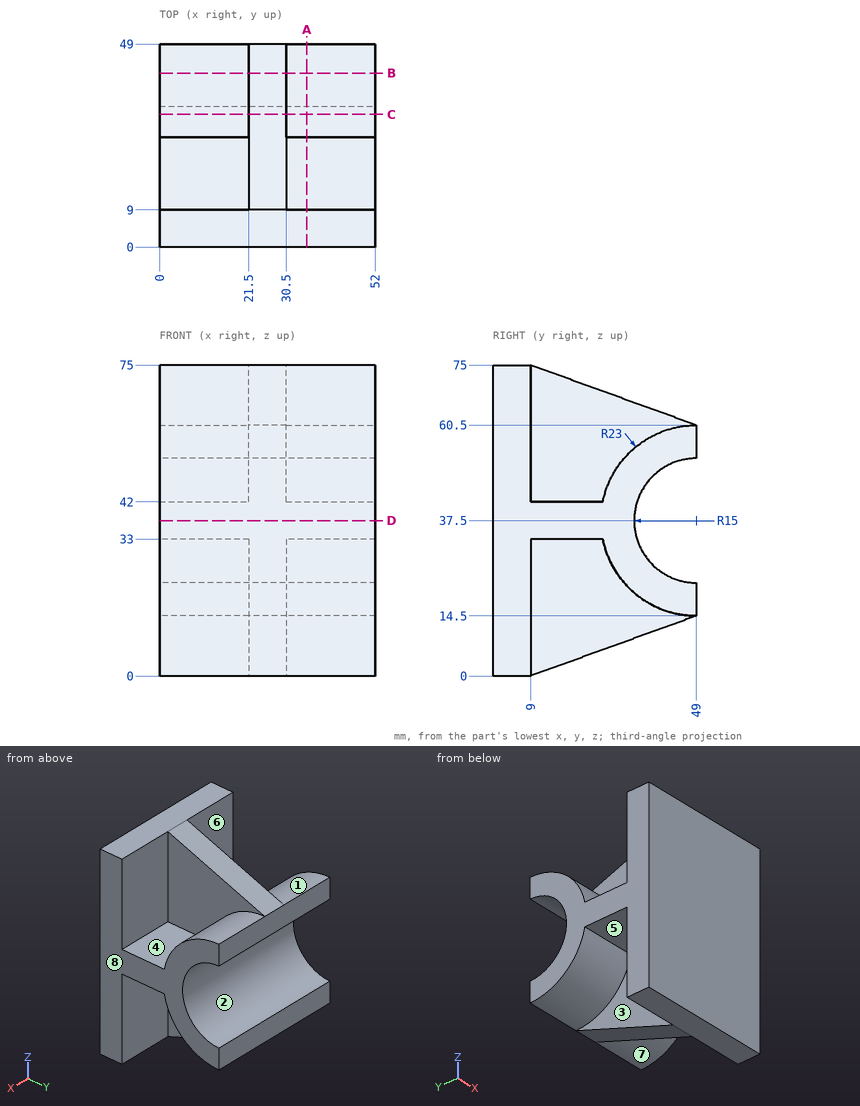
Can you work these out from the drawing? Everything is in mm from the part's minimum corner. A direction names the side the tool comes from. Coordinates: 2 decimals unless noted, no trailing zeros. Loops run counter-clockwise (first coordinate to the right, second up) from the corner with the lowest first, then second, coordinate; pieces in that order, holes last.
1) Imagine slicing it at D-D on z = 37.5. List the corners of the cut face in (x, y) for me, plus the area to 3 significant figures.
2) I need wall thicknesses on probe 1 along Z at (x, y) = (38, 16); probe 2 along Y at (x, z) = (5.5, 67.5); probe 3 along X at (y, z) = (13.5, 43.5). Which ranges of each line are inside material? Lowest first, please.
3) Which directions (+Z, -Z, +X, -X, +Y, -Y) give clear straight access to the entire face, cutting with the end or side of a thin tool? Please do the marked faces 4, 5, 6, 7 and 8.
4) For pin 1 (3 mm diameter, centred on x = 36.5, z = 30.5, fed in from +Y); pin 2 (10 mm diameter, centred on x = 21, y = 44, fed in from +Z); pin 3 (8.5 mm diameter, centred on x = 10, y = 18, fed in from -Z), each with a flat end and sliding along its axis, tell me the tip position at first contact or that it passes through.
5) Imagine slicing it at B-B on y = 42. List the corners of the cut face in (x, z) for me, plus the area to 3 significant figures.
6) Thinking about a two-plate mould opening in Z: for the marked faces 1, 2 and 3, which applies, pulls with the +Z half, pulls with the -Z half, needs draft (parallel to the pull), parting line crosses it, or undercut?
7) Imagine slicing it at A-A on x = 35.5. List the corners of the cut face in (y, z) for me.
8) Imagine slicing it at C-C on y = 32. List the corners of the cut face in (x, z) for me, plus the area to 3 significant figures.
Completed:
1. outline: (0, 0) - (52, 0) - (52, 34) - (0, 34) - close
1. area: 1,770 mm2
2. probe 1: z = 33 to 42
2. probe 2: y = 0 to 9
2. probe 3: x = 21.5 to 30.5
3. face 4: +Z, +X
3. face 5: -Z, -X
3. face 6: +Z, -X
3. face 7: -Z, +X
3. face 8: +Z, -Z, +X, +Y, -Y
4. pin 1: stops at y = 36.64
4. pin 2: stops at z = 64.12
4. pin 3: stops at z = 33
5. outline: (0, 15.59) - (21.5, 15.59) - (21.5, 11.96) - (30.5, 11.96) - (30.5, 15.59) - (52, 15.59) - (52, 24.23) - (0, 24.23) - close; (0, 50.77) - (52, 50.77) - (52, 59.41) - (30.5, 59.41) - (30.5, 63.04) - (21.5, 63.04) - (21.5, 59.41) - (0, 59.41) - close
5. area: 964 mm2
6. face 1: pulls with the +Z half
6. face 2: undercut
6. face 3: needs draft
7. outline: (0, 0) - (9, 0) - (9, 33) - (26.44, 33) arc R23 ccw to (49, 14.5) - (49, 22.5) arc R15 cw to (49, 52.5) - (49, 60.5) arc R23 ccw to (26.44, 42) - (9, 42) - (9, 75) - (0, 75) - close
8. outline: (0, 22.01) - (21.5, 22.01) - (21.5, 8.34) - (30.5, 8.34) - (30.5, 22.01) - (52, 22.01) - (52, 52.99) - (30.5, 52.99) - (30.5, 66.66) - (21.5, 66.66) - (21.5, 52.99) - (0, 52.99) - close
8. area: 1,860 mm2
